Part model, mm, in its own coordinate system. Face numbers are marked on the shaded views. Coordinates: 2 decimals unless noted, no trailing zeros. Use a Markdown table: item, result. Add a question column.
Q1. Pin check, flat tips, straight feed: pin 1 Ø9 at (x, z) = (3280, 1459.5) entering from +Y; pin 2 Ø1.1 at (x, z) = (3259.5, 1250) entering from -Y; pin 3 Ø24 at (x, y) = (3277, 4311.5) entering from -Z. Stop position of each tip, or through.
Q2. Wall check: L1, parallel to Z at x = 3261, y = 4481; L2, parallel to X at y = 4075.5, z = 949; L3, parallel to X at y = 4087, z = 406.5. Give the ranges that are in metal, low to high. Write a range as from..to.
Q3. Mould opens along Z. For the marked faces 1, 2 and 3 say: released by +Z, released by -Z, zero draft, split by the parting line, or undercut.
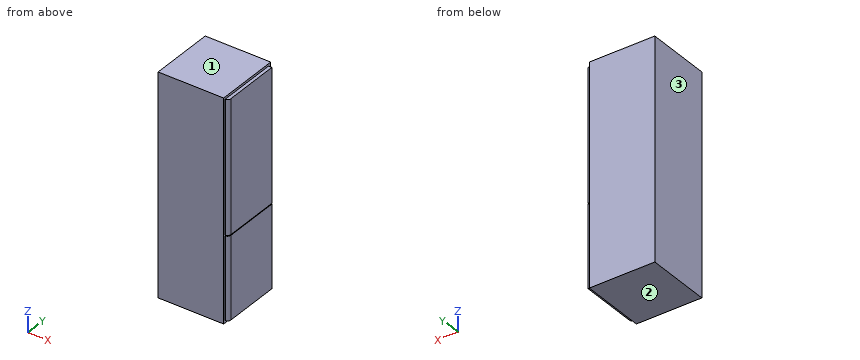
from build123d import *

# Parameters (mm, degrees)
SKETCH627_W             = 597
SKETCH627_H             = 600
PAD300_DEPTH            = 2011
SKETCH628_W             = 550
SKETCH628_H             = 1210
PAD301_DEPTH            = 30
FILLET211_R             = 29
SKETCH629_W             = 550
SKETCH629_H             = 754
PAD302_DEPTH            = 30
FILLET212_R             = 29
BODY127_PLACEMENT_ANGLE = 90


with BuildPart() as part:
    # Sketch627 → Pad300 (new body)
    with BuildSketch(Plane.XY):
        with Locations((298.5, 300)):
            Rectangle(SKETCH627_W, SKETCH627_H)
    extrude(amount=PAD300_DEPTH)

    # Sketch628 (on Face1 of Pad300) → Pad301 (join)
    with BuildSketch(Plane.XZ):
        with Locations((295, 1385)):
            Rectangle(SKETCH628_W, SKETCH628_H)
    extrude(amount=PAD301_DEPTH)

    # Fillet211
    fillet211_edges = [part.edges().sort_by_distance(p)[0] for p in [
        (20, -30, 1385),
    ]]
    fillet(fillet211_edges, radius=FILLET211_R)

    # Sketch629 (on Face4 of Fillet211) → Pad302 (join)
    with BuildSketch(Plane.XZ):
        with Locations((295, 397)):
            Rectangle(SKETCH629_W, SKETCH629_H)
    extrude(amount=PAD302_DEPTH)

    # Fillet212
    fillet212_edges = [part.edges().sort_by_distance(p)[0] for p in [
        (20, -30, 397),
    ]]
    fillet(fillet212_edges, radius=FILLET212_R)


with BuildPart() as part_1:
    # Body127 placement: moved
    add(part.part.moved(Location((3259, 4046, 15))).rotate(Axis((3259, 4046, 15), (0, 0, 1)), BODY127_PLACEMENT_ANGLE))


solid = part_1.part
Recorded:
| question | item | result |
|---|---|---|
| 1 | pin 1 | y = 4616 |
| 1 | pin 2 | y = 4046 |
| 1 | pin 3 | z = 35 |
| 2 | L1 | 35..789, 795..2005 |
| 2 | L2 | 2659..3281.47 |
| 2 | L3 | 2659..3287.87 |
| 3 | face 1 | released by +Z |
| 3 | face 2 | released by -Z |
| 3 | face 3 | zero draft |
